Can you work these out from the model? Positions are in its coordinate system, mm. A direction names the side the tool comes from. Coordinates: 2 decimals unless noted, no trailing zeros. Order: outer loops, then holes, each group sorted by start corner. A loop starts at its lowest first (then second) coordinate and runs counter-clockwise, first axis right, second up. Notation, with made-up numbers: M 41.5,68.5 L 81.5,68.5 A23 ccw 81.5,92.5 Z; hole C 28.25,23.5 d2. An arc over 180 degrees is marked long. Answer as CSV lines item,"result". Start each with the question number.
1. If we section it at C-C (y = -51): List the corners of the cut face in (x, z) for me, plus the area to 3 significant figures.
2. On a 3-axis mill with a long thin cutter (end or side, diameter ignored), from which of +Z, -Z, +X, -X, +Y, -Y can I reach the whole of each face in a straight line? I mean faces 1 (the face through (-3.905, -69.174, 0.867)), 2 (the face through (20, 0, 0)), 3 (the face through (-0.1, 13.5, -20.3)), 4 (the face through (-18, 0, 18)), 5 (the face through (-15, -23.5, -15)). Say none if no direction works.
3. I need wall thicknesses on line 1 along Z through (x, y) = (15.5, -1.5); line 2 along X through (y, z) = (-4, 6.5). Which ranges of each line are inside material? Lowest first, please. Write a range as from..to.
4. If we section it at A-A (y = -12.5): List the corners of the cut face in (x, z) for me.
5. If we section it at B-B (z = 0): List the corners of the cut face in (x, y) for me.
6. If we section it at D-D (y = -64): List the corners of the cut face in (x, z) for me.
7. If we mould it in two halves opening along X, with no side actions, what happens to faces 6 (the face through (10.275, -56.328, -11.092)), 7 (the face through (19, -18, -19)), 8 (the face through (-19, 18, 19))? For each: released by +X, released by -X, zero draft, split by the parting line, or undercut.
8. Will these pins go through, and if not, where does the flat tip stop? pin 1 (4 mm diameter, centred on x = -10, y = 4.5, fed in from +Z); pin 2 (0.8 mm diameter, centred on x = -10, z = -10, fed in from -Y); pin 3 (3 mm diameter, centred on x = 9.9, z = 9.9, fed in from -Y).
```python
from build123d import *

# Parameters (mm, degrees)
SKETCH1_W               = 42
SKETCH1_H               = 42
BOSS_EXTRUDE1_DEPTH     = 23.5
CUT_EXTRUDE1_START      = -10
SKETCH2_W               = 42
SKETCH2_H               = 42
SKETCH2_W_2             = 40
SKETCH2_H_2             = 40
CUT_EXTRUDE1_DEPTH      = 27
CHAMFER1_SIZE           = 4
CUT_EXTRUDE2_DEPTH      = 56.596762496
CUT_EXTRUDE2_DEPTH_BACK = 56.596762496
SKETCH4_R               = 1.25
BOSS_EXTRUDE2_DEPTH     = 4.8
SKETCH6_R               = 18
BOSS_EXTRUDE3_DEPTH     = 30
SKETCH7_R               = 1.25
CUT_EXTRUDE3_DEPTH      = 4
SKETCH8_R               = 11
BOSS_EXTRUDE4_DEPTH     = 2
SKETCH9_R               = 4
BOSS_EXTRUDE5_DEPTH     = 18
BOSS_EXTRUDE6_START     = -15
BOSS_EXTRUDE6_DEPTH     = 15


with BuildPart() as part:
    # Sketch1 → Boss-Extrude1 (new, symmetric)
    with BuildSketch(Plane(origin=(0, 0, 0), x_dir=(1, 0, 0), z_dir=(0, 1, 0))):
        Rectangle(SKETCH1_W, SKETCH1_H)
    extrude(amount=BOSS_EXTRUDE1_DEPTH, both=True)

    # Sketch2 → Cut-Extrude1 (cut)
    with BuildSketch(Plane(origin=(0, 23.5, 0), x_dir=(1, 0, 0), z_dir=(0, 1, 0)).offset(CUT_EXTRUDE1_START)):
        Rectangle(SKETCH2_W, SKETCH2_H)
        Rectangle(SKETCH2_W_2, SKETCH2_H_2, mode=Mode.SUBTRACT)
    extrude(amount=-CUT_EXTRUDE1_DEPTH, mode=Mode.SUBTRACT)

    # Chamfer1
    chamfer1_edges = [part.edges().sort_by_distance(p)[0] for p in [
        (-21, -18.5, -21),
        (21, -18.5, -21),
        (21, -18.5, 21),
        (-21, -18.5, 21),
        (20, 0, -20),
        (20, 0, 20),
        (-20, 0, 20),
        (-20, 0, -20),
        (-21, 18.5, -21),
        (21, 18.5, -21),
        (21, 18.5, 21),
        (-21, 18.5, 21),
    ]]
    chamfer(chamfer1_edges, length=CHAMFER1_SIZE)

    # Sketch4 → Cut-Extrude2 (cut, two sides: drawn at the far end of the back side and taken through both)
    with BuildSketch(Plane(origin=(0, 23.5, 0), x_dir=(1, 0, 0), z_dir=(0, 1, 0)).offset(-CUT_EXTRUDE2_DEPTH_BACK)):
        with Locations(Location((15.5, 15.5, 0), (0, 0, 270))):
            Circle(SKETCH4_R)
        with Locations(Location((15.5, -15.5, 0), (0, 0, 270))):
            Circle(SKETCH4_R)
        with Locations(Location((-15.5, -15.5, 0), (0, 0, 270))):
            Circle(SKETCH4_R)
        with Locations(Location((-15.5, 15.5, 0), (0, 0, 270))):
            Circle(SKETCH4_R)
    extrude(amount=CUT_EXTRUDE2_DEPTH + CUT_EXTRUDE2_DEPTH_BACK, mode=Mode.SUBTRACT)

    # Sketch5 → Boss-Extrude2 (add)
    with BuildSketch(Plane.XZ.offset(23.5)):
        Polygon((-20, 16), (-16, 20), (16, 20), (20, 16), (20, -16), (16, -20), (-16, -20), (-20, -16), align=None)
    extrude(amount=BOSS_EXTRUDE2_DEPTH)

    # Sketch6 → Boss-Extrude3 (add)
    with BuildSketch(Plane.XZ.offset(28.3)):
        with Locations(Location((0, 0, 0), (0, 0, 270))):
            Circle(SKETCH6_R)
    extrude(amount=BOSS_EXTRUDE3_DEPTH)

    # Sketch7 → Cut-Extrude3 (cut)
    with BuildSketch(Plane.XZ.offset(58.3)):
        with Locations(Location((-9.899494937, 9.899494937, 0), (0, 0, 270))):
            Circle(SKETCH7_R)
        with Locations(Location((9.899494937, 9.899494937, 0), (0, 0, 270))):
            Circle(SKETCH7_R)
        with Locations(Location((9.899494937, -9.899494937, 0), (0, 0, 270))):
            Circle(SKETCH7_R)
        with Locations(Location((-9.899494937, -9.899494937, 0), (0, 0, 270))):
            Circle(SKETCH7_R)
    extrude(amount=-CUT_EXTRUDE3_DEPTH, mode=Mode.SUBTRACT)

    # Sketch8 → Boss-Extrude4 (add)
    with BuildSketch(Plane.XZ.offset(58.3)):
        with Locations(Location((0, 0, 0), (0, 0, 270))):
            Circle(SKETCH8_R)
    extrude(amount=BOSS_EXTRUDE4_DEPTH)

    # Sketch9 → Boss-Extrude5 (add)
    with BuildSketch(Plane.XZ.offset(60.3)):
        with Locations(Location((0, 0, 0), (0, 0, 270))):
            Circle(SKETCH9_R)
    extrude(amount=BOSS_EXTRUDE5_DEPTH)

    # Sketch10 → Boss-Extrude6 (add)
    with BuildSketch(Plane.XZ.offset(78.3).offset(BOSS_EXTRUDE6_START)):
        with BuildLine():
            Line((-2.645751311, 3), (2.645751311, 3))
            ThreePointArc((2.645751311, 3), (0, 4), (-2.645751311, 3))
        make_face()
    extrude(amount=BOSS_EXTRUDE6_DEPTH)


solid = part.part
```
Solved:
1,outline,"C 0,0 d36"
1,area,"1,020 mm²"
2,face 1,"-Y"
2,face 2,"+Z, -Z, +X"
2,face 3,"none"
2,face 4,"+Z, -X"
2,face 5,"+Y"
3,line 1,"-20..-16.75, -14.25..14.25, 16.75..20"
3,line 2,"-20..20"
4,outline,"M -20,-16 L -16,-20 L 16,-20 L 20,-16 L 20,16 L 16,20 L -16,20 L -20,16 Z; hole C -15.5,-15.5 d2.5; hole C -15.5,15.5 d2.5; hole C 15.5,-15.5 d2.5; hole C 15.5,15.5 d2.5"
5,outline,"M -21,-23.5 L -20,-23.5 L -20,-28.3 L -18,-28.3 L -18,-58.3 L -11,-58.3 L -11,-60.3 L -4,-60.3 L -4,-78.3 L 4,-78.3 L 4,-60.3 L 11,-60.3 L 11,-58.3 L 18,-58.3 L 18,-28.3 L 20,-28.3 L 20,-23.5 L 21,-23.5 L 21,-13.5 L 20,-13.5 L 20,13.5 L 21,13.5 L 21,23.5 L -21,23.5 L -21,13.5 L -20,13.5 L -20,-13.5 L -21,-13.5 Z"
6,outline,"C 0,0 d8"
7,face 6,"undercut"
7,face 7,"released by +X"
7,face 8,"released by -X"
8,pin 1,"z = 20"
8,pin 2,"y = -54.3"
8,pin 3,"y = -58.3"
